from build123d import *

# Parameters (mm, degrees)
SKETCH1_R           = 2.5
BOSS_EXTRUDE1_DEPTH = 5
CUT_EXTRUDE1_START  = -2
SKETCH2_R           = 2
SKETCH2_R_2         = 1
CUT_EXTRUDE1_DEPTH  = 11.051970793
SKETCH2_2_R         = 1
CUT_EXTRUDE2_DEPTH  = 13.051970793


with BuildPart() as part:
    # Sketch1 → Boss-Extrude1 (new body)
    with BuildSketch(Plane.XY):
        with BuildLine():
            Line((-7.5, 4), (7.5, 4))
            Line((7.5, 4), (3.321799308, -2.228373702))
            ThreePointArc((3.321799308, -2.228373702), (0, -4), (-3.321799308, -2.228373702))
            Line((-3.321799308, -2.228373702), (-7.5, 4))
        make_face()
        Circle(SKETCH1_R, mode=Mode.SUBTRACT)
    extrude(amount=BOSS_EXTRUDE1_DEPTH)

    # Sketch2 → Cut-Extrude1 (cut, through all)
    # profile 1 of 2: a face of its own
    with BuildSketch(Plane(origin=(0, 4, 0), x_dir=(1, 0, 0), z_dir=(0, 1, 0)).offset(CUT_EXTRUDE1_START)):
        with Locations((-5.4, -2.5)):
            Circle(SKETCH2_R)
        with Locations((-5.4, -2.5)):
            Circle(SKETCH2_R_2, mode=Mode.SUBTRACT)
    # profile 2 of 2: a face of its own
    with BuildSketch(Plane(origin=(0, 4, 0), x_dir=(1, 0, 0), z_dir=(0, 1, 0)).offset(CUT_EXTRUDE1_START)):
        with Locations((5.4, -2.5)):
            Circle(SKETCH2_R)
        with Locations((5.4, -2.5)):
            Circle(SKETCH2_R_2, mode=Mode.SUBTRACT)
    extrude(amount=-CUT_EXTRUDE1_DEPTH, mode=Mode.SUBTRACT)

    # Sketch2_2 → Cut-Extrude2 (cut, through all)
    with BuildSketch(Plane(origin=(0, 4, 0), x_dir=(1, 0, 0), z_dir=(0, 1, 0))):
        with Locations(Location((-5.4, -2.5, 0), (0, 0, 270))):
            Circle(SKETCH2_2_R)
        with Locations(Location((5.4, -2.5, 0), (0, 0, 270))):
            Circle(SKETCH2_2_R)
    extrude(amount=-CUT_EXTRUDE2_DEPTH, mode=Mode.SUBTRACT)


solid = part.part
Build history of the part. All positions in model axes, mm. Coordinates: 2 decimals unless noted, no trailing zeros. Order: outer loops, then holes, each group sorted by start corner. A loop starts at its lowest first (then second) coordinate and runs counter-clockwise, first axis right, second up. Notation, with made-up numbers: M -12,83 L 26,83 A34 cw 26,114 Z; hole C 54.5,39 d5. An arc over 180 degrees is marked long. One line per question, with ' | ' between items. Start each with the question number.
Q1. Flat gauge pins, fed straight in: pin 1 Ø3 at (x, z) = (-4.5, 2.5) entering from -Y; pin 2 Ø2.5 at (x, z) = (-5.4, 2.5) entering from -Y; pin 3 Ø3 at (x, z) = (4, 1.5) entering from -Y. Where does each tip first touch, or does it go through?
Q2. Saw through at A-A (x = 0). List the corners of the cut face in (y, z), then the cut area to 3 significant figures.
Q3. Saw through at B-B (z = 2.5). List the corners of the cut face in (x, y).
Q4. Two-plate mould, pull along Z, no slides. Class faces 1 (the face through (-4.41, 3.01, 2.37)), 2 (the face through (0, 3, 5)), 3 (the face through (0, 3, 0)): +Z half, -Z half, draft (parallel to the pull), parting line (faces both ways), or undercut.
Q5. Saw through at C-C (y = 0). List the corners of the cut face in (x, z).
Q6. Saw through at D-D (z = 3.8). List the corners of the cut face in (x, y), then the cut area to 3 significant figures.
Q7. Probe L1, parallel to Z at x = 5.4, y = 2.55; L2, parallel to X at y = -0.15, z = 2.5; L3, parallel to Y at x = -0.5, z = 2.85. List the from-to ranges inside material, lowest first. Write a range as from..to.
Check values:
1) pin 1: stops at y = -2.65 | pin 2: stops at y = 2 | pin 3: stops at y = -3.12
2) outline: M -4,0 L -2.5,0 L -2.5,5 L -4,5 Z; M 2.5,0 L 4,0 L 4,5 L 2.5,5 Z | area: 15.0 mm2
3) outline: M -7.5,4 L -6.4,2.36 L -6.4,4 Z; M -4.4,2 L -3.4,2 L -3.4,-2.11 L -3.32,-2.23 A4 ccw 3.32,-2.23 L 3.4,-2.11 L 3.4,2 L 4.4,2 L 4.4,4 L -4.4,4 Z; M 6.4,2.36 L 7.5,4 L 6.4,4 Z; hole C 0,0 d5
4) face 1: undercut | face 2: +Z half | face 3: -Z half
5) outline: M -4.82,0 L -2.5,0 L -2.5,5 L -4.82,5 L -4.82,4.41 A2 cw -4.82,0.59 Z; M 2.5,0 L 4.82,0 L 4.82,0.59 A2 cw 4.82,4.41 L 4.82,5 L 2.5,5 Z
6) outline: M -7.5,4 L -6.16,2 L -3.88,2 L -3.88,-1.4 L -3.32,-2.23 A4 ccw 3.32,-2.23 L 3.88,-1.4 L 3.88,2 L 6.16,2 L 7.5,4 Z; hole C 0,0 d5 | area: 48.3 mm2
7) L1: z = 0..1.5, 3.5..5 | L2: x = -3.4..-2.5, 2.5..3.4 | L3: y = -3.97..-2.45, 2.45..4
